Verification items for the finished model (mm, model axes). Give positions to 0.01 mm unless a question says otherwise; leave off trailing zeros. Order: outer loops, then holes, each group sorted by start corner. A loop starts at its lowest first (then second) coordinate and runs counter-clockwise, first axis right, second up.
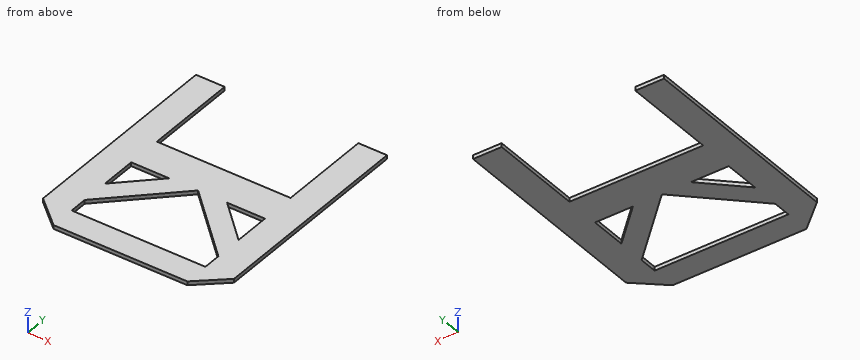
from build123d import *

# Parameters (mm, degrees)
F1_DEPTH = 1.2


with BuildPart() as f1:
    # F0 (on Top) → F1 (new body)
    with BuildSketch(Plane.XY):
        Polygon((20.888254, -36.877837), (-20.888254, -36.877837), (-20.888254, -31.238344), (-20.888254, -22.505017), (-20.888254, -11.076983), (-20.888254, 0), (-20.888254, 29.34467), (-29.831249, 29.34467), (-29.831249, -36.877837), (-20.888254, -44.694535), (0, -44.694535), (20.888254, -44.694535), (29.831249, -36.877837), (29.831249, 29.34467), (20.888254, 29.34467), (20.888254, 0), (20.888254, -11.076983), (20.888254, -22.505017), (20.888254, -31.238344), align=None)
        Polygon((-9.048197, -11.076983), (0, -11.076983), (9.048197, -11.076983), (20.888254, -11.076983), (20.888254, 0), (-20.888254, 0), (-20.888254, -11.076983), align=None)
        Polygon((-20.888254, -22.505017), (-20.888254, -31.238344), (0, -11.076983), (-9.048197, -11.076983), align=None)
        Polygon((0, -11.076983), (20.888254, -31.238344), (20.888254, -22.505017), (9.048197, -11.076983), align=None)
    extrude(amount=F1_DEPTH)


solid = f1.part
(1) Section check D-D, the plane x = 10.5. Enter the section's corners in (y, z), then the cut area to 3 significant figures.
Solved:
outline: (-44.69, 0) - (-36.88, 0) - (-36.88, 1.2) - (-44.69, 1.2) - close; (-21.21, 0) - (-12.48, 0) - (-12.48, 1.2) - (-21.21, 1.2) - close; (-11.08, 0) - (0, 0) - (0, 1.2) - (-11.08, 1.2) - close
area: 33.2 mm2
(2) Section check C-C, the plane x = -5. Enter the section's corners in (y, z).
Solved:
outline: (-44.69, 0) - (-36.88, 0) - (-36.88, 1.2) - (-44.69, 1.2) - close; (-15.9, 0) - (0, 0) - (0, 1.2) - (-15.9, 1.2) - close
(3) Scan lines: line 1 (Y direction, x = 16, z = 0.1); line 2 (X direction, y = -21, z = 0.9); line 3 (X direction, y = -32.5, z = 0.75). Record each from-to range of solid material in increasing order.
Solved:
line 1: y = -44.69 to -36.88, -26.52 to -17.79, -11.08 to 0
line 2: x = -29.83 to -20.89, -19.33 to -10.28, 10.28 to 19.33, 20.89 to 29.83
line 3: x = -29.83 to -20.89, 20.89 to 29.83
(4) Section check B-B, the plane z = 0.75. Enter the section's corners in (x, y), then the cut area to 3 significant figures.
Solved:
outline: (-29.83, -36.88) - (-20.89, -44.69) - (20.89, -44.69) - (29.83, -36.88) - (29.83, 29.34) - (20.89, 29.34) - (20.89, 0) - (-20.89, 0) - (-20.89, 29.34) - (-29.83, 29.34) - close; hole (-20.89, -36.88) - (20.89, -36.88) - (20.89, -31.24) - (0, -11.08) - (-20.89, -31.24) - close; hole (-20.89, -22.51) - (-9.05, -11.08) - (-20.89, -11.08) - close; hole (9.05, -11.08) - (20.89, -22.51) - (20.89, -11.08) - close
area: 2,330 mm2
(5) Go/stop test with flat-tipped pins: pin 1 (5 mm diameter, centred on x = 10, y = -14, fed in from -Z); pin 2 (0.6 mm diameter, centred on x = -8, z = 0.5, fed in from +Y). Record where each tip stops, or that it passes through.
Solved:
pin 1: stops at z = 0
pin 2: stops at y = 0
(6) Section check A-A, the plane y = 16. Enter the section's corners in (x, z), then the cut area to 3 significant figures.
Solved:
outline: (-29.83, 0) - (-20.89, 0) - (-20.89, 1.2) - (-29.83, 1.2) - close; (20.89, 0) - (29.83, 0) - (29.83, 1.2) - (20.89, 1.2) - close
area: 21.5 mm2
